Can you work these out from the drawing? Everything is in mm from the part's minimum corner. A direction names the side the tool comes from. Coordinates: 2 decimals unless noted, no trailing zeros. Loops run counter-clockwise (first coordinate to the right, second up) from the corner with the lowest first, then second, coordinate; pieces in that order, holes last. Notation, with made-up numbers: (-30, 35.5) -> (3, 35.5) arc R31 cw to (3, 61.5) -> close; hole circle Ø8 at (51.5, 73). An arc over 180 degrees is marked (long way). Put each result on its own line as item: value. Start each with the question number.
Item 1: If we section it at C-C on y = 9.5: Please give me the cut outline in (x, z).
Item 2: Will these pins go through, and if not, where does the flat tip stop? P1, Ø12, axis at y = 22.5, z = 4.5, coming from the +X side; P2, Ø1, axis at x = 16.5, z = 20.5, coming from the +Y side.
Item 3: If we section it at A-A on z = 16.25: Please give me the cut outline in (x, y).
Item 4: For the marked faces 4 and 5, which set-ups out of +Z, -Z, +X, -X, +Y, -Y let a thin tool reach every point of the face, with its end or its side?
Item 5: Please list where these lines run through material, in increasing order: L1, parallel to Z at x = 8, y = 5.75; L2, parallel to Y at x = 14.25, z = 13.25. Write a range as from..to.
Item 6: If we section it at B-B on x = 10.5: Please give me the cut outline in (y, z).
Item 7: We'd pull the mould along Z, two halves only. Please class the marked faces 1, 2 and 3: pulls with the +Z half, pulls with the -Z half, needs draft (parallel to the pull), parting line crosses it, or undercut.
Item 8: If we section it at D-D on x = 14: Please give me the cut outline in (y, z), plus the area to 3 significant figures.
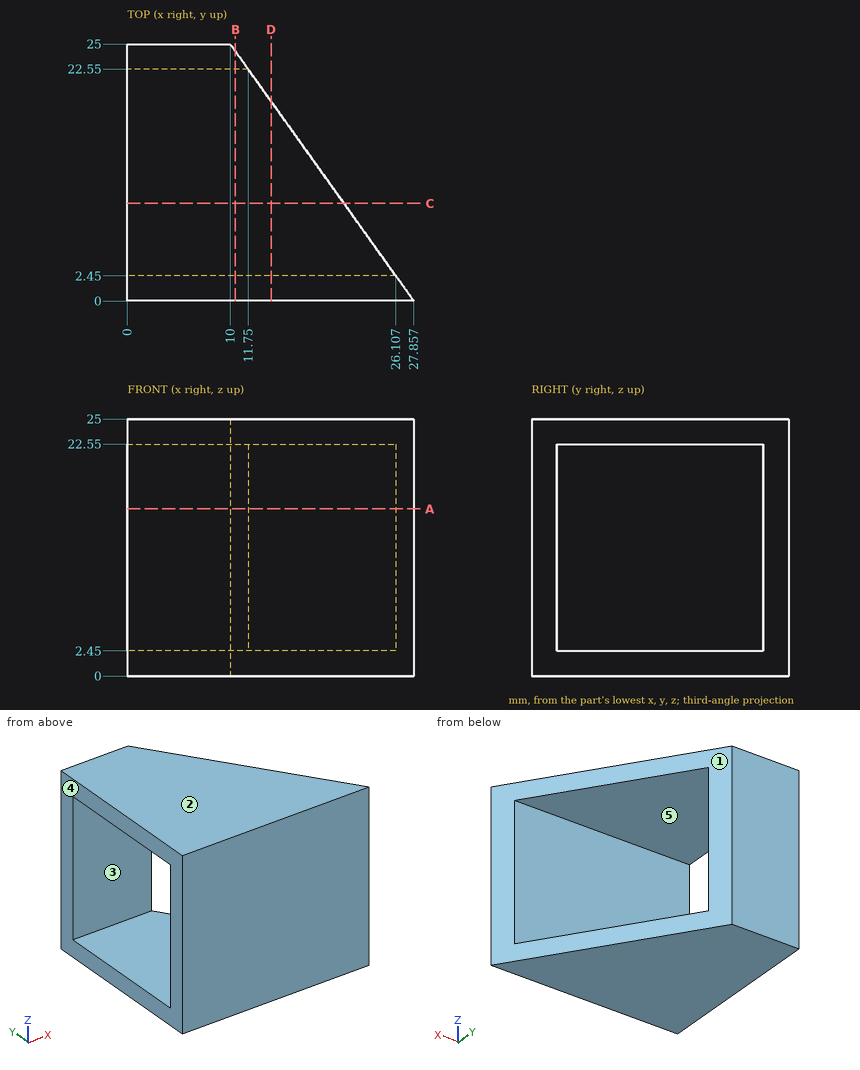
Solutions:
1. outline: (0, 0) -> (21.07, 0) -> (21.07, 2.45) -> (0, 2.45) -> close; (0, 22.55) -> (21.07, 22.55) -> (21.07, 25) -> (0, 25) -> close
2. P1: x = 15.81
2. P2: y = 2.45
3. outline: (0, 0) -> (27.86, 0) -> (26.11, 2.45) -> (0, 2.45) -> close; (0, 22.55) -> (11.75, 22.55) -> (10, 25) -> (0, 25) -> close
4. face 4: +Z, -Z, -X, +Y, -Y
4. face 5: +X, -X
5. L1: 0..2.45, 22.55..25
5. L2: 0..2.45
6. outline: (0, 0) -> (24.3, 0) -> (24.3, 25) -> (0, 25) -> close; hole (2.45, 2.45) -> (22.55, 2.45) -> (22.55, 22.55) -> (2.45, 22.55) -> close
7. face 1: needs draft
7. face 2: pulls with the +Z half
7. face 3: undercut
8. outline: (0, 0) -> (19.4, 0) -> (19.4, 2.45) -> (2.45, 2.45) -> (2.45, 22.55) -> (19.4, 22.55) -> (19.4, 25) -> (0, 25) -> close
8. area: 144 mm^2
